The listing builds one solid part. Answer for the finished solid, in the listing's coordinates (mm). Coordinates: 2 decimals unless noted, no trailing zeros. Order: outer loops, then holes, each group sorted by start corner. A loop starts at its lowest first (then second) coordinate and runs counter-clockwise, first axis right, second up. Notation, with made-up numbers: M -8.5,33.5 L 3.5,33.5 A24 cw 3.5,57.5 Z; hole C 49,-9 d7. An arc over 180 degrees is marked long. One line per item, written item: value. Start each with the question number.
Q1. Each of these flat-tipped pins is pushed along its axis until it touches: pin 1 Ø1.4 at (x, y) = (-87, 2.5) entering from +Z; pin 2 Ø3 at (x, y) = (-59, 2.5) entering from +Z; pin 3 Ø0.9 at (x, y) = (-85, 5.5) entering from +Z. Where does it stop, or does it pass through?
Q2. The part is cut by section A-A on x = -61.5. Give the vertices of the cut face in (y, z).
Q3. Straight lines are drawn through the part: line 1 along X through (y, z) = (5, 25); line 2 along Z through (x, y) = (17.5, 1.5); line 3 along Z through (x, y) = (-41, 4.25). For each, find the intervals that lie inside material, in ascending order. Write a range as [from, to].
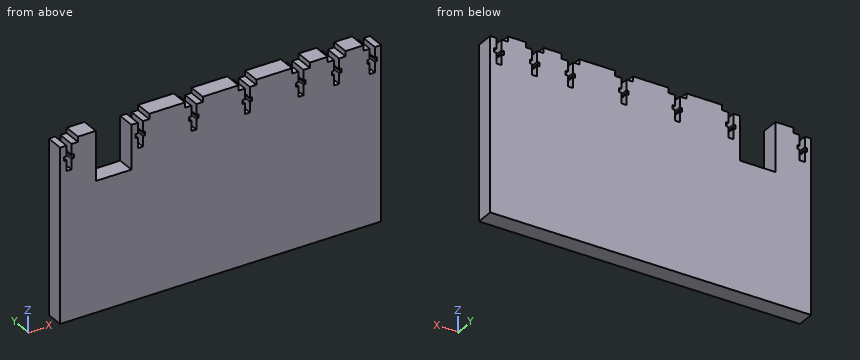
```python
from build123d import *

# Parameters (mm, degrees)
SKETCH1_W           = 10
SKETCH1_H           = 2.907263933
SKETCH1_W_2         = 20
BOSS_EXTRUDE1_DEPTH = 10
SKETCH3_W           = 2.85
SKETCH3_H           = 14
SKETCH3_W_2         = 5.35
SKETCH3_H_2         = 2.2
CUT_EXTRUDE1_DEPTH  = 10


with BuildPart() as part:
    # Sketch1 → Boss-Extrude1 (new body)
    with BuildSketch(Plane(origin=(0, 0, 0), x_dir=(1, 0, 0), z_dir=(0, 1, 0))):
        Polygon((80, -48.454398885), (90, -48.454398885), (90, 48.454398885), (-90, 48.454398885), (-90, -48.454398885), (-80, -48.454398885), (-70, -48.454398885), (-70, -23.839564252), (-50, -23.839564252), (-50, -48.454398885), (-40, -48.454398885), (-20, -48.454398885), (-10, -48.454398885), (10, -48.454398885), (20, -48.454398885), (40, -48.454398885), (50, -48.454398885), (60, -48.454398885), (70, -48.454398885), align=None)
        with Locations((-75, -49.908030852)):
            Rectangle(SKETCH1_W, SKETCH1_H)
        with Locations((-30, -49.908030852)):
            Rectangle(SKETCH1_W_2, SKETCH1_H)
        with Locations((0, -49.908030852)):
            Rectangle(SKETCH1_W_2, SKETCH1_H)
        with Locations((30, -49.908030852)):
            Rectangle(SKETCH1_W_2, SKETCH1_H)
        with Locations((55, -49.908030852)):
            Rectangle(SKETCH1_W, SKETCH1_H)
        with Locations((75, -49.908030852)):
            Rectangle(SKETCH1_W, SKETCH1_H)
    extrude(amount=BOSS_EXTRUDE1_DEPTH)

    # Sketch3 → Cut-Extrude1 (cut)
    with BuildSketch(Plane(origin=(0, 10, 0), x_dir=(1, 0, 0), z_dir=(0, 1, 0))):
        with Locations((-85, -41.454398885)):
            Rectangle(SKETCH3_W, SKETCH3_H)
        with Locations((-85, -41.454398885)):
            Rectangle(SKETCH3_W_2, SKETCH3_H_2)
        with Locations((-45, -41.454398885)):
            Rectangle(SKETCH3_W, SKETCH3_H)
        with Locations((-45, -41.454398885)):
            Rectangle(SKETCH3_W_2, SKETCH3_H_2)
        with Locations((-15, -41.454398885)):
            Rectangle(SKETCH3_W, SKETCH3_H)
        with Locations((-15, -41.454398885)):
            Rectangle(SKETCH3_W_2, SKETCH3_H_2)
        with Locations((15, -41.454398885)):
            Rectangle(SKETCH3_W, SKETCH3_H)
        with Locations((15, -41.454398885)):
            Rectangle(SKETCH3_W_2, SKETCH3_H_2)
        with Locations((45, -41.454398885)):
            Rectangle(SKETCH3_W, SKETCH3_H)
        with Locations((45, -41.454398885)):
            Rectangle(SKETCH3_W_2, SKETCH3_H_2)
        with Locations((65, -41.454398885)):
            Rectangle(SKETCH3_W, SKETCH3_H)
        with Locations((65, -41.454398885)):
            Rectangle(SKETCH3_W_2, SKETCH3_H_2)
        with Locations((85, -41.454398885)):
            Rectangle(SKETCH3_W, SKETCH3_H)
        with Locations((85, -41.454398885)):
            Rectangle(SKETCH3_W_2, SKETCH3_H_2)
    extrude(amount=-CUT_EXTRUDE1_DEPTH, mode=Mode.SUBTRACT)


solid = part.part
```
Output:
1. pin 1: stops at z = 48.45
1. pin 2: stops at z = 23.84
1. pin 3: stops at z = 34.45
2. outline: M 0,-48.45 L 10,-48.45 L 10,23.84 L 0,23.84 Z
3. line 1: x = [-90, -70], [-50, 90]
3. line 2: z = [-48.45, 40.35], [42.55, 48.45]
3. line 3: z = [-48.45, 48.45]
